```python
from build123d import *

# Parameters (mm, degrees)
SKETCH1_W           = 60
SKETCH1_H           = 20
BOSS_EXTRUDE1_DEPTH = 1
SKETCH2_W           = 58
SKETCH2_H           = 18
BOSS_EXTRUDE2_DEPTH = 1
SKETCH4_R           = 2.5
SKETCH4_W           = 1
SKETCH4_H           = 14
CUT_EXTRUDE2_DEPTH  = 4
CHAMFER2_START      = 7.522135998
CHAMFER2_2_DEPTH    = 13
CHAMFER2_START_2    = -23
CHAMFER2_3_DEPTH    = 10.5
CHAMFER2_START_3    = -29
CHAMFER2_4_DEPTH    = 7
CHAMFER2_START_4    = -7
CHAMFER2_5_DEPTH    = 14
CHAMFER2_START_5    = -5.5
CHAMFER2_6_DEPTH    = 11
CHAMFER2_START_6    = -9
CHAMFER2_7_DEPTH    = 18
CHAMFER2_8_DEPTH    = 2
CHAMFER2_START_7    = 7
CHAMFER2_9_DEPTH    = 2


with BuildPart() as part:
    # Sketch1 → Boss-Extrude1 (new body)
    with BuildSketch(Plane.XY):
        Rectangle(SKETCH1_W, SKETCH1_H)
    extrude(amount=BOSS_EXTRUDE1_DEPTH)

    # Sketch2 → Boss-Extrude2 (add)
    with BuildSketch(Plane.XY.offset(1)):
        Rectangle(SKETCH2_W, SKETCH2_H)
    extrude(amount=BOSS_EXTRUDE2_DEPTH)

    # Sketch4 → Cut-Extrude2 (cut)
    with BuildSketch(Plane(origin=(0, 0, 0), x_dir=(-1, 0, 0), z_dir=(0, 0, -1))):
        with Locations((-4, 0)):
            Circle(SKETCH4_R)
        Polygon((13.5, -5.5), (23, -5.5), (23, -7), (29, -7), (29, -5.5), (29, 5.5), (29, 7), (23, 7), (23, 5.5), (13.5, 5.5), align=None)
        with Locations((-20.022135998, 0)):
            Rectangle(SKETCH4_W, SKETCH4_H)
        with Locations((-17.022135998, 0)):
            Rectangle(SKETCH4_W, SKETCH4_H)
        with Locations((-14.022135998, 0)):
            Rectangle(SKETCH4_W, SKETCH4_H)
        with Locations((-11.022135998, 0)):
            Rectangle(SKETCH4_W, SKETCH4_H)
        with Locations((-8.022135998, 0)):
            Rectangle(SKETCH4_W, SKETCH4_H)
    extrude(amount=-CUT_EXTRUDE2_DEPTH, mode=Mode.SUBTRACT)

    # Chamfer2: read off the stored shape, not the designer's step
    # Chamfer2 outline → Chamfer2 (revolve, cut)
    with BuildSketch(Plane(origin=(4, 0, 0), x_dir=(1, 0, 0), z_dir=(0, -1, 0))):
        Polygon((3.5, 0), (2.5, 2), (2.5, 0), align=None)
    revolve(axis=Axis((4, 0, 0), (0, 0, 1)), mode=Mode.SUBTRACT)

    # Chamfer2 2 outline → Chamfer2 2 (cut)
    with BuildSketch(Plane.YZ.offset(CHAMFER2_START)):
        Polygon((7, 2), (7, 0), (8, 0), align=None)
        Polygon((5.5, 2), (5.5, 0), (6.5, 0), align=None)
        Polygon((-5.5, 2), (-6.5, 0), (-5.5, 0), align=None)
        Polygon((-7, 2), (-8, 0), (-7, 0), align=None)
    extrude(amount=CHAMFER2_2_DEPTH, mode=Mode.SUBTRACT)

    # Chamfer2 3 outline → Chamfer2 3 (cut)
    with BuildSketch(Plane.YZ.offset(CHAMFER2_START_2)):
        Polygon((5.5, 2), (5.5, 0), (6.5, 0), align=None)
        Polygon((-5.5, 2), (-6.5, 0), (-5.5, 0), align=None)
    extrude(amount=CHAMFER2_3_DEPTH, mode=Mode.SUBTRACT)

    # Chamfer2 4 outline → Chamfer2 4 (cut)
    with BuildSketch(Plane.YZ.offset(CHAMFER2_START_3)):
        Polygon((7, 2), (7, 0), (8, 0), align=None)
        Polygon((-7, 2), (-8, 0), (-7, 0), align=None)
    extrude(amount=CHAMFER2_4_DEPTH, mode=Mode.SUBTRACT)

    # Chamfer2 5 outline → Chamfer2 5 (cut)
    with BuildSketch(Plane(origin=(0, 0, 0), x_dir=(1, 0, 0), z_dir=(0, 1, 0)).offset(CHAMFER2_START_4)):
        Polygon((18.522135998, 0), (19.522135998, -2), (19.522135998, 0), align=None)
        Polygon((17.522135998, -2), (18.522135998, 0), (17.522135998, 0), align=None)
        Polygon((15.522135998, 0), (16.522135998, -2), (16.522135998, 0), align=None)
        Polygon((14.522135998, -2), (15.522135998, 0), (14.522135998, 0), align=None)
        Polygon((12.522135998, 0), (13.522135998, -2), (13.522135998, 0), align=None)
        Polygon((11.522135998, -2), (12.522135998, 0), (11.522135998, 0), align=None)
        Polygon((9.522135998, 0), (10.522135998, -2), (10.522135998, 0), align=None)
        Polygon((8.522135998, -2), (9.522135998, 0), (8.522135998, 0), align=None)
        Polygon((-23, -2), (-22, 0), (-23, 0), align=None)
    extrude(amount=CHAMFER2_5_DEPTH, mode=Mode.SUBTRACT)

    # Chamfer2 6 outline → Chamfer2 6 (cut)
    with BuildSketch(Plane(origin=(0, 0, 0), x_dir=(1, 0, 0), z_dir=(0, 1, 0)).offset(CHAMFER2_START_5)):
        Polygon((-13.5, -2), (-12.5, 0), (-13.5, 0), align=None)
    extrude(amount=CHAMFER2_6_DEPTH, mode=Mode.SUBTRACT)

    # Chamfer2 7 outline → Chamfer2 7 (add)
    with BuildSketch(Plane(origin=(0, 0, 0), x_dir=(1, 0, 0), z_dir=(0, 1, 0)).offset(CHAMFER2_START_6)):
        Polygon((17.522135998, -2), (19.522135998, -2), (18.522135998, 0), align=None)
        Polygon((14.522135998, -2), (16.522135998, -2), (15.522135998, 0), align=None)
        Polygon((11.522135998, -2), (13.522135998, -2), (12.522135998, 0), align=None)
        Polygon((8.522135998, -2), (10.522135998, -2), (9.522135998, 0), align=None)
        Polygon((-13.5, -2), (-12.5, -2), (-12.5, 0), align=None)
    extrude(amount=CHAMFER2_7_DEPTH)

    # Chamfer2 8 outline → Chamfer2 8 (add)
    with BuildSketch(Plane(origin=(0, 0, 0), x_dir=(1, 0, 0), z_dir=(0, 1, 0)).offset(CHAMFER2_START_6)):
        Polygon((-23, -2), (-22, -2), (-22, 0), align=None)
    extrude(amount=CHAMFER2_8_DEPTH)

    # Chamfer2 9 outline → Chamfer2 9 (add)
    with BuildSketch(Plane(origin=(0, 0, 0), x_dir=(1, 0, 0), z_dir=(0, 1, 0)).offset(CHAMFER2_START_7)):
        Polygon((-23, -2), (-22, -2), (-22, 0), align=None)
    extrude(amount=CHAMFER2_9_DEPTH)


solid = part.part
```
Here's how the part is built. I have some questions about the finished solid (model axes, mm). A direction names the side the tool comes from. Coordinates: 2 decimals unless noted, no trailing zeros. Order: outer loops, then holes, each group sorted by start corner. A loop starts at its lowest first (then second) coordinate and runs counter-clockwise, first axis right, second up.
1) Imagine slicing it at A-A on x = 4. List the corners of the cut face in (y, z) for me.
2) We'd pull the mould along X, two halves only. Please class faces 1 (the face through (13.029, -0.112, 1.014)), 2 (the face through (-0.4, -10, 0.5)), 3 (the face through (-29, -8.2, 1.5)): +X half, -X half, draft (parallel to the pull), parting line (faces both ways), or undercut.
3) Which directions (+Z, -Z, +X, -X, +Y, -Y) give clear straight access to the entire face, cutting with the end or side of a thin tool? Please do faces 4 (the face through (14, 7.6, 0.8)), 5 (the face through (29, -0.1, 1.5)), 6 (the face through (-0.4, -9, 1.5)), 7 (the face through (0, 0, 0)).
4) I need wall thicknesses on line 1 (X direction, y = 3.25, z = 1.1); line 2 (X direction, y = 5.75, z = 1.3); line 3 (Y direction, x = -14.5, z = 0.55) (3 decimals). Which ranges of each line are inside material? Lowest first, please.
5) Imagine slicing it at B-B on y = 0. State how many separate pieces and enclosed holes the cut face has, and give its area (3 significant figures).
6) Will these pins go through, and if not, where does the flat tip stop? pin 1 (0.8 mm diameter, centred on x = -13.5, z = 1.5, fed in from -Y); pin 2 (0.8 mm diameter, centred on y = 3, z = 1.5, fed in from +X); pin 3 (10 mm diameter, centred on x = 2, y = 5.5, fed in from -Z); pin 4 (0.5 mm diameter, centred on x = 11.5, z = 1.5, fed in from +Y).
7) Imagine slicing it at C-C on y = -4.5. List the corners of the cut face in (x, z) for me, and give its area (3 significant figures).
Response values:
1. outline: (-10, 0) - (-3.5, 0) - (-2.5, 2) - (-9, 2) - (-9, 1) - (-10, 1) - close; (2.5, 2) - (3.5, 0) - (10, 0) - (10, 1) - (9, 1) - (9, 2) - close
2. face 1: undercut
2. face 2: draft
2. face 3: -X half
3. face 4: -Z
3. face 5: +Z, +X, +Y, -Y
3. face 6: +Z, +X, -X, -Y
3. face 7: -Z, +X, -X, +Y, -Y
4. line 1: x = -13.05 to 7.52, 8.97 to 10.07, 11.97 to 13.07, 14.97 to 16.07, 17.97 to 19.07, 20.52 to 29
4. line 2: x = -13.15 to 7.52, 8.87 to 10.17, 11.87 to 13.17, 14.87 to 16.17, 17.87 to 19.17, 20.52 to 29
4. line 3: y = -10 to -6.225, 6.225 to 10
5. separate pieces: 8
5. enclosed holes: 0
5. area: 56.0 mm2
6. pin 1: stops at y = -9
6. pin 2: stops at x = 29
6. pin 3: stops at z = 0
6. pin 4: stops at y = 9
7. outline: (-30, 0) - (-29, 0) - (-29, 1) - (-30, 1) - close; (-13.5, 2) - (-12.5, 0) - (7.52, 0) - (7.52, 2) - close; (8.52, 2) - (9.52, 0) - (10.52, 2) - close; (11.52, 2) - (12.52, 0) - (13.52, 2) - close; (14.52, 2) - (15.52, 0) - (16.52, 2) - close; (17.52, 2) - (18.52, 0) - (19.52, 2) - close; (20.52, 0) - (30, 0) - (30, 1) - (29, 1) - (29, 2) - (20.52, 2) - close
7. area: 68.0 mm2
